Read the model definition and answer for the solid it produces. Units are mm, in the model's axes. A direction names the side the tool comes from. Round coordinates to 2 decimals unless told otherwise and drop trailing zeros. Order: outer loops, then holes, each group sorted by start corner. A loop starts at its lowest first (then second) coordinate and runs counter-clockwise, first axis right, second up. Notation, with made-up numbers: (-2.75, 71) - (1.25, 71) arc R23 ccw to (1.25, 100) - close; hole circle Ø4 at (54, 67). An arc over 180 degrees is marked (long way). Answer as a JSON object with one key per item and string values. Group by question number.
Q1. The mould has two halves that part along X. Classify faces 1 (the flat face through (-10, -6, 76.2)), 2 (the cylindrical face through (-11.4, 13.8, 2)), 3 (the cylindrical face through (23.846, -7.509, 1.972)): pulls with the +X half, pulls with the -X half, needs draft (parallel to the pull), parting line crosses it, or undercut.
Q2. Consider line 1 (Y direction, x = 0, z = 33); line 2 (X direction, y = -0.5, z = 50); line 3 (Z direction, x = -1, y = 19). Determine where each line is inside the solid, lowest interval first.
Q3. A tool of negligible diameter and unlimited length cuts with its end or side. For faces 4 (the cylindrical face through (10.78, -3.4, 37.57)), 5 (the flat face through (11, 11, 4)), from which of +Z, -Z, +X, -X, +Y, -Y can it reach the whole face along a straight path? Write none if from no direction.
Q4. A cutting plane is placed at A-A on x = 0. Determine the outline of the cut face in (y, z), and give its area (3 significant figures).
Q5. Given pin 1 Ø5 at (y, z) = (0, 60.325) entering from -X; pin 2 Ø4 at (x, y) = (12.49, -15.62) entering from -Z; pin 3 Ø2 at (x, z) = (-11.5, 22.5) entering from -Y; pin 4 Ø2 at (x, z) = (-7.5, 34) entering from -Y, each flat-ended and moving along its own axis, determine where each tip first touches the part or whether it passes through.
Q6. A cutting plane is placed at D-D on x = 7. Determine the outline of the cut face in (y, z).
Q7. A cutting plane is placed at B-B on y = 0. Determine the outline of the cut face in (x, z), and give its area (3 significant figures).
Q8. A cutting plane is placed at C-C on z = 10. Determine the outline of the cut face in (x, y).
Autodesk Fusion 360 part; units mm, degrees
sketch "Sketch1" plane through (0, 0, 0) normal (0, 0, 1) x (1, 0, 0)
  circle A0 centre (0, 0) radius 11.303
  circle A1 centre (0, 0) radius 25
  circle A2 centre (0, 0) radius 15.24
  circle A3 centre (-12.4939, 15.6174) radius 2.1209
  line L0 (0, 25) -> (0, -25) construction
  line L1 (-25, 0) -> (25, 0) construction
  line L2 (-25, 0) -> (25, 0) construction
  circle A4 centre (12.4939, 15.6174) radius 2.1209
  circle A5 centre (-12.4939, -15.6174) radius 2.1209
  circle A6 centre (12.4939, -15.6174) radius 2.1209
  dimension "d1" = 22.606
  dimension "d2" = 30.48
  dimension "d3" = 50
  dimension "d4" = 20
  dimension "d5" = 4.2418
extrude "Extrude1" add sketch "Sketch1" along normal blind 4 contours A1
extrude "Extrude2" add sketch "Sketch1" along normal blind 76.2 contours A2
sketch "Sketch2" plane through (0, 0, 0) normal (1, 0, 0) x (0, 1, 0)
  circle A0 centre (0, 60.325) radius 2.1209
  dimension "d10" = 4.2418
  dimension "d11" = 60.325
extrude "Extrude3" cut sketch "Sketch2" along normal through all and the other way through all
Result set:
{
 "1": {"face 1": "needs draft", "face 2": "undercut", "face 3": "parting line crosses it"},
 "2": {"line 1": "y = -15.24 to -11.3, 11.3 to 15.24", "line 2": "x = -15.23 to -11.29, 11.29 to 15.23", "line 3": "z = 0 to 4"},
 "3": {"face 4": "+Z, -Z", "face 5": "+Z"},
 "4": {"outline": "(-25, 0) - (-11.3, 0) - (-11.3, 76.2) - (-15.24, 76.2) - (-15.24, 4) - (-25, 4) - close; (11.3, 0) - (25, 0) - (25, 4) - (15.24, 4) - (15.24, 76.2) - (11.3, 76.2) - close", "area": "678 mm²"},
 "5": {"pin 1": "stops at x = -15.24", "pin 2": "passes through", "pin 3": "stops at y = -11.05", "pin 4": "stops at y = -13.78"},
 "6": {"outline": "(-24, 0) - (-8.87, 0) - (-8.87, 76.2) - (-13.54, 76.2) - (-13.54, 4) - (-24, 4) - close; (8.87, 0) - (24, 0) - (24, 4) - (13.54, 4) - (13.54, 76.2) - (8.87, 76.2) - close"},
 "7": {"outline": "(-25, 0) - (-11.3, 0) - (-11.3, 58.2) - (-15.24, 58.2) - (-15.24, 4) - (-25, 4) - close; (-15.24, 62.45) - (-11.3, 62.45) - (-11.3, 76.2) - (-15.24, 76.2) - close; (11.3, 0) - (25, 0) - (25, 4) - (15.24, 4) - (15.24, 58.2) - (11.3, 58.2) - close; (11.3, 62.45) - (15.24, 62.45) - (15.24, 76.2) - (11.3, 76.2) - close", "area": "645 mm²"},
 "8": {"outline": "circle Ø30.48 at (0, 0); hole circle Ø22.61 at (0, 0)"}
}
